Check sheet for the modelled part. Datum: model origin and axes. Units: mm. Coordinates: 2 decimals unless noted, no trailing zeros. Loops run counter-clockwise (first coordinate to the right, second up) from the corner with the lowest first, then second, coordinate; pieces in that order, holes last. Notation, with made-up numbers: (23, 76) -> (73, 76) arc R27 ccw to (73, 100) -> close; hole circle Ø1 at (35, -21.75). An arc over 180 degrees is marked (long way). Use CSV: the item, a comma, the result in double quotes.
```python
from build123d import *

# Parameters (mm, degrees)
SKETCH1_W           = 11
SKETCH1_H           = 18
SKETCH1_W_2         = 5
SKETCH1_H_2         = 11
BOSS_EXTRUDE1_DEPTH = 4
BOSS_EXTRUDE2_DEPTH = 5
SKETCH3_R           = 1.248430758
CUT_EXTRUDE1_DEPTH  = 5
FILLET1_R           = 1
FILLET3_R           = 2
FILLET4_R           = 9
CUT_EXTRUDE2_DEPTH  = 10
CHAMFER1_SIZE       = 1


with BuildPart() as part:
    # Sketch1 → Boss-Extrude1 (new body)
    with BuildSketch(Plane(origin=(0, 0, 0), x_dir=(1, 0, 0), z_dir=(0, 1, 0))):
        with Locations((-2.740875912, 16.357664234)):
            Rectangle(SKETCH1_W, SKETCH1_H)
        with Locations((-5.740875912, 30.857664234)):
            Rectangle(SKETCH1_W_2, SKETCH1_H_2)
    boss_extrude1 = extrude(amount=BOSS_EXTRUDE1_DEPTH)

    # Sketch2 → Boss-Extrude2 (add)
    with BuildSketch(Plane(origin=(-3.240875912, 0, 0), x_dir=(0, 0, -1), z_dir=(1, 0, 0))):
        with BuildLine():
            Line((34.537911903, 0), (25.357664234, 0))
            Line((25.357664234, 0), (25.357664234, -12.192130501))
            Line((25.357664234, -12.192130501), (34.537911903, -12.192130501))
            Line((34.537911903, -12.192130501), (34.537911903, -7.165523267))
            ThreePointArc((34.537911903, -7.165523267), (33.357664234, -5.7), (34.537911903, -4.234476733))
            Line((34.537911903, -4.234476733), (34.537911903, 0))
        make_face()
        with BuildLine():
            Line((36.357664234, 0), (34.537911903, 0))
            Line((34.537911903, 0), (34.537911903, -4.234476733))
            ThreePointArc((34.537911903, -4.234476733), (35.798507341, -4.531747353), (36.357664234, -5.7))
            ThreePointArc((36.357664234, -5.7), (35.798507341, -6.868252647), (34.537911903, -7.165523267))
            Line((34.537911903, -7.165523267), (34.537911903, -12.192130501))
            ThreePointArc((34.537911903, -12.192130501), (41.293121094, -6.613725887), (36.357664234, 0.62455532))
            Line((36.357664234, 0.62455532), (36.357664234, 0))
        make_face()
    boss_extrude2 = extrude(amount=-BOSS_EXTRUDE2_DEPTH)

    # Mirror1: Boss-Extrude1, Boss-Extrude2 across plane
    add(boss_extrude1.mirror(Plane(origin=(-8.240875912, 4, 0), x_dir=(0, 0, 1), z_dir=(1, 0, 0))))
    add(boss_extrude2.mirror(Plane(origin=(-8.240875912, 4, 0), x_dir=(0, 0, 1), z_dir=(1, 0, 0))))

    # Sketch3 → Cut-Extrude1 (cut)
    with BuildSketch(Plane(origin=(0, 4, 0), x_dir=(1, 0, 0), z_dir=(0, 1, 0))):
        with Locations(Location((-2.240875912, 13.357664234, 0), (0, 0, 270))):
            Circle(SKETCH3_R)
        with Locations(Location((-14.240875912, 13.357664234, 0), (0, 0, 270))):
            Circle(SKETCH3_R)
    extrude(amount=-CUT_EXTRUDE1_DEPTH, mode=Mode.SUBTRACT)

    # Fillet1
    fillet1_edges = [part.edges().sort_by_distance(p)[0] for p in [
        (-0.240875912, 4, -25.357664234),
        (-3.240875912, -4.234476733, -35.177416564),
        (-8.240875912, 4, -7.357664234),
        (-19.240875912, 4, -16.357664234),
        (-16.240875912, 4, -25.357664234),
        (2.759124088, 4, -16.357664234),
        (-13.240875912, -4.234476733, -35.177416564),
    ]]
    fillet(fillet1_edges, radius=FILLET1_R)

    # Fillet3
    fillet3_edges = [part.edges().sort_by_distance(p)[0] for p in [
        (-8.240875912, 0, -25.357664234),
    ]]
    fillet(fillet3_edges, radius=FILLET3_R)

    # Fillet4
    fillet4_edges = [part.edges().sort_by_distance(p)[0] for p in [
        (-8.240875912, -12.192130501, -25.357664234),
    ]]
    fillet(fillet4_edges, radius=FILLET4_R)

    # Sketch4 → Cut-Extrude2 (cut)
    with BuildSketch(Plane.ZY.offset(13.240875912)):
        Polygon((-36.357664234, 0.62455532), (-24.357664234, 4), (-36.357664234, 4), align=None)
    extrude(amount=-CUT_EXTRUDE2_DEPTH, mode=Mode.SUBTRACT)

    # Chamfer1
    chamfer1_edges = [part.edges().sort_by_distance(p)[0] for p in [
        (-2.240875912, 4, -14.606094992),
        (-14.240875912, 4, -14.606094992),
    ]]
    chamfer(chamfer1_edges, length=CHAMFER1_SIZE)


solid = part.part
```
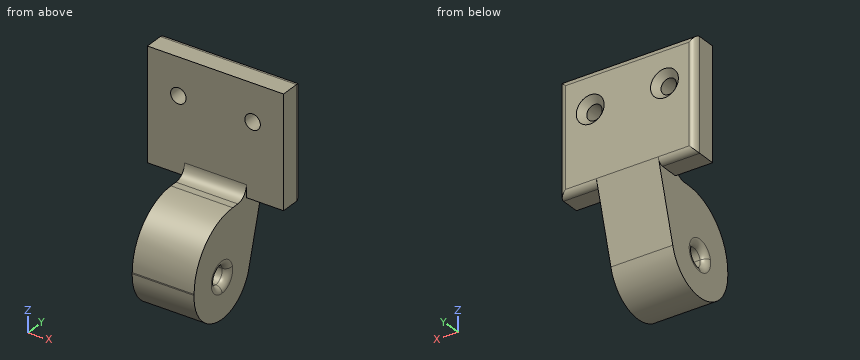
1) Thickness scan on line 1 along X through (y, z) = (-6, -26); line 2 along Z through (x, y) = (-15.75, 2); line 3 along Z through (x, y) = (-10.25, -5.5). Record the ranges inside material, lowest first. Write a range as from..to.
Answer below:
line 1,"x = -13.24..-3.24"
line 2,"z = -25.36..-7.36"
line 3,"z = -41.35..-36.34, -33.37..-25.66"
2) Cross-section at A-A on x = -9. Record the boundary of the cut face in (y, z).
Answer below:
outline,"(-12.19, -34.54) arc R6.5 ccw to (0.62, -36.36) -> (4, -24.36) -> (4, -8.36) arc R1 ccw to (3, -7.36) -> (0, -7.36) -> (0, -23.36) arc R2 cw to (-2, -25.36) -> (-3.19, -25.36) arc R9 ccw to (-12.19, -34.36) -> close; hole circle Ø3 at (-5.7, -34.86)"
3) Cross-section at D-D on z = -19. Record the boundary of the cut face in (x, y), and give its area (3 significant figures).
Answer below:
outline,"(-19.24, 0) -> (2.76, 0) -> (2.76, 3) arc R1 ccw to (1.76, 4) -> (-18.24, 4) arc R1 ccw to (-19.24, 3) -> close"
area,"87.6 mm²"
4) Cross-section at C-C on z = -13. Give the number of separate pieces and of enclosed holes in the cut face, and give its area (3 significant figures).
Answer below:
separate pieces,"3"
enclosed holes,"0"
area,"66.4 mm²"
5) Go/stop test with flat-tipped pins: pin 1 Ø5 at (x, y) = (-14, -8.5) entering from -Z; pin 2 Ø8 at (y, z) = (-7.5, -23) entering from +X; pin 3 Ø0.9 at (x, y) = (-1, 1.5) entering from -Z. Record where each tip stops, or that it passes through.
Answer below:
pin 1,"stops at z = -41.34"
pin 2,"stops at x = -3.24"
pin 3,"stops at z = -25.36"
6) Cross-section at B-B on y = 1. Record the boundary of the cut face in (x, z).
Answer below:
outline,"(-19.24, -25.36) -> (-13.24, -25.36) -> (-13.24, -35.02) -> (-3.24, -35.02) -> (-3.24, -25.36) -> (2.76, -25.36) -> (2.76, -7.36) -> (-19.24, -7.36) -> close; hole circle Ø2.5 at (-14.24, -13.36); hole circle Ø2.5 at (-2.24, -13.36)"
